```python
from build123d import *

# Parameters (mm, degrees)
BOSS_EXTRU_1_DEPTH      = 10
ESQUISSE2_R             = 1
ENL_V_MAT_EXTRU_1_DEPTH = 20


with BuildPart() as part:
    # Esquisse1 → Boss.-Extru.1 (new body)
    with BuildSketch(Plane.XY):
        Polygon((-99.151357472, 118.130872671), (-101.873142366, 116.869172631), (-80.844808358, 71.506091068), (-78.123023465, 72.767791109), (-83.169823626, 83.654930684), (-79.540777101, 85.337197404), (-74.49397694, 74.450057829), (-71.772192046, 75.71175787), (-92.800526053, 121.074839432), (-95.522310947, 119.813139392), (-90.475510785, 108.925999817), (-94.10455731, 107.243733096), align=None)
    extrude(amount=BOSS_EXTRU_1_DEPTH)

    # Esquisse2 → Enlèv. mat.-Extru.1 (cut)
    with BuildSketch(Plane(origin=(-39.261124148, -18.199734313, 0), x_dir=(0, 0, 1), z_dir=(-0.9072616312569982, -0.42056668014583676, 0))):
        with BuildLine():
            ThreePointArc((0, 143.875365486), (1.464466094, 147.410899392), (5, 148.875365486))
            Line((5, 148.875365486), (0, 148.875365486))
            Line((0, 148.875365486), (0, 143.875365486))
        make_face()
        with BuildLine():
            ThreePointArc((5, 148.875365486), (8.535533906, 147.410899392), (10, 143.875365486))
            Line((10, 143.875365486), (10, 148.875365486))
            Line((10, 148.875365486), (5, 148.875365486))
        make_face()
        with Locations(Location((5, 143.875365486, 0), (0, 0, 270))):
            Circle(ESQUISSE2_R)
        with BuildLine():
            Line((10, 98.875365486), (10, 103.875365486))
            ThreePointArc((10, 103.875365486), (8.535533906, 100.33983158), (5, 98.875365486))
            Line((5, 98.875365486), (10, 98.875365486))
        make_face()
        with BuildLine():
            Line((0, 98.875365486), (5, 98.875365486))
            ThreePointArc((5, 98.875365486), (1.464466094, 100.33983158), (0, 103.875365486))
            Line((0, 103.875365486), (0, 98.875365486))
        make_face()
        with Locations(Location((5, 103.875365486, 0), (0, 0, 270))):
            Circle(ESQUISSE2_R)
    extrude(amount=-ENL_V_MAT_EXTRU_1_DEPTH, mode=Mode.SUBTRACT)


solid = part.part
```
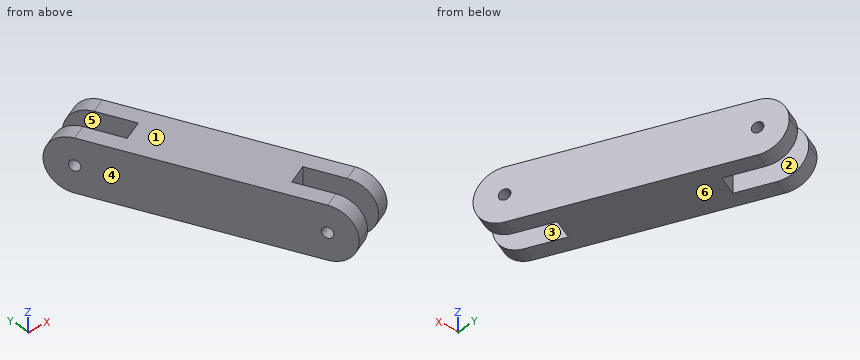
Geometry check sheet. Reference: the model listing, model coordinates, mm. Face numbers are marked on the shaded views. A direction names the side the tool comes from. Coordinates: 2 decimals unless noted, no trailing zeros. Write each loop counter-clockwise with the first axis right and the second up, starting at its lowest first coordinate (ties: lowest second). Pieces come first, ordered by that corner, then holes. Notation, with made-up numbers: (-7, 8) -> (40, 8) arc R22 ccw to (40, 40) -> close; hole circle Ø8 at (-37, -14.5). An arc over 180 degrees is marked (long way). Use CSV: the item, a comma, the result in double quotes. Start each with the question number.
Item 1: Cross-section at D-D, the plane z = 9.5. Record the cut outline in (x, y), plus the area to 3 significant figures.
Item 2: Mould release check, pull along Y, two halves, no side actions. Record for the marked faces 1, 2, 3 and 4: released by +Y, released by -Y, zero draft, split by the parting line, or undercut.
Item 3: Thickness scan on line 1 (Y direction, x = -95, z = 3.5); line 2 (Y direction, x = -93, z = 2.5); line 3 (X direction, y = 113, z = 1.25). Record the ranges inside material, lowest first.
Item 4: Cross-section at C-C, the plane x = -86. Record the cut outline in (y, z), plus the area to 3 significant figures.
Item 5: Depth check by flat-ended pin: pin 1 Ø1 at (y, z) = (94.5, 5.5) entering from +X; pin 2 Ø2 at (x, z) = (-91.5, 7.5) entering from +Y. Enter the tip coordinate at first touch or a pass-through.
Item 6: Cross-section at B-B, the plane y = 82. Record the cut outline in (x, z), plus the area to 3 significant figures.
Item 7: Set-up check for the marked faces 5 and 6: record each of +Z, -Z, +X, -X, +Y, -Y from which the full face is reachable in a straight line by a thin tool's end or side.
Item 8: Cross-section at A-A, the plane z = 3. Record the cut outline in (x, y).
Answers:
1,outline,"(-100.69, 114.31) -> (-82.03, 74.07) -> (-79.31, 75.33) -> (-83.17, 83.65) -> (-79.54, 85.34) -> (-75.68, 77.01) -> (-72.96, 78.27) -> (-91.61, 118.52) -> (-94.34, 117.25) -> (-90.48, 108.93) -> (-94.1, 107.24) -> (-97.97, 115.57) -> close"
1,area,"370 mm^2"
2,face 1,"zero draft"
2,face 2,"undercut"
2,face 3,"undercut"
2,face 4,"released by -Y"
3,line 1,"102.04 to 109.18, 118.69 to 119.8"
3,line 2,"97.73 to 107.76, 114.37 to 120.24"
3,line 3,"-100.08 to -96.77, -92.36 to -89.06"
4,outline,"(82.63, 0) -> (106.4, 0) -> (106.4, 10) -> (82.63, 10) -> close"
4,area,"238 mm^2"
5,pin 1,"x = -80.25"
5,pin 2,"y = 120.43"
6,outline,"(-85.71, 0) -> (-82.4, 0) -> (-82.4, 10) -> (-85.71, 10) -> close; (-77.99, 0) -> (-74.69, 0) -> (-74.69, 10) -> (-77.99, 10) -> close"
6,area,"66.1 mm^2"
7,face 5,"+Z, -Z"
7,face 6,"-Z, +X, -X, +Y, -Y"
8,outline,"(-101.7, 116.49) -> (-81.02, 71.88) -> (-78.3, 73.15) -> (-83.17, 83.65) -> (-79.54, 85.34) -> (-74.67, 74.83) -> (-71.95, 76.09) -> (-92.62, 120.7) -> (-95.35, 119.43) -> (-90.48, 108.93) -> (-94.1, 107.24) -> (-98.98, 117.75) -> close"
